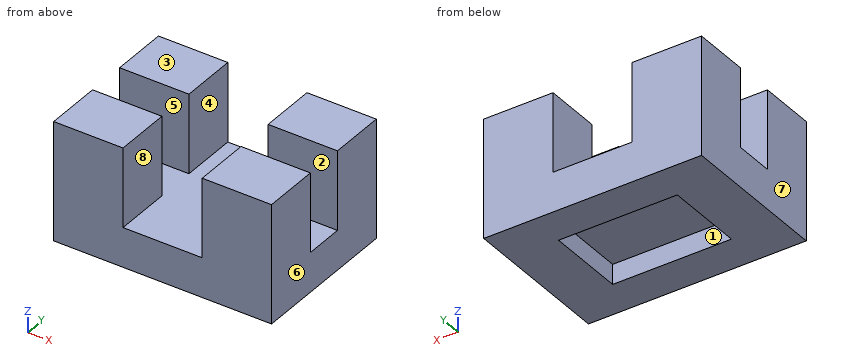
```python
from build123d import *

# Parameters (mm, degrees)
F0_W     = 17.4752
F0_H     = 12.2936
F1_DEPTH = 9.525
F2_W     = 6.35
F2_H     = 12.2936
F3_DEPTH = 6.35
F4_W     = 17.4752
F4_H     = 3.175
F5_DEPTH = 6.35
F6_W     = 9.525
F6_H     = 6.35
F7_DEPTH = 1.6002


with BuildPart() as f1:
    # F0 (on Top) → F1 (new body)
    with BuildSketch(Plane.XY):
        Rectangle(F0_W, F0_H)
    extrude(amount=F1_DEPTH)

    # F2 (on face) → F3 (cut)
    with BuildSketch(Plane.XY.offset(9.525)):
        Rectangle(F2_W, F2_H)
    extrude(amount=-F3_DEPTH, mode=Mode.SUBTRACT)

    # F4 (on face) → F5 (cut)
    with BuildSketch(Plane.XY.offset(9.525)):
        Rectangle(F4_W, F4_H)
    extrude(amount=-F5_DEPTH, mode=Mode.SUBTRACT)

    # F6 (on face) → F7 (cut)
    with BuildSketch(Plane(origin=(0, 0, 0), x_dir=(1, 0, 0), z_dir=(0, 0, -1))):
        Rectangle(F6_W, F6_H)
    extrude(amount=-F7_DEPTH, mode=Mode.SUBTRACT)


solid = f1.part
```
Geometry: final body of the model. Coordinates: model frame, mm. Face numbers are marked on the shaded views. A direction names the side the tool comes from. Round coordinates to 2 decimals unless told otherwise and drop trailing zeros. Write each loop counter-clockwise with the first axis right and the second up, starting at its lowest first coordinate (ties: lowest second). Pieces come first, ordered by that corner, then holes.
Item 1: Set-up query: the marked faces 1, 2, 3 and 4. Return all of +Z, -Z, +X, -X, +Y, -Y with unobstructed straight access to the full face (end or side cutting, diameter ignored); none if empty.
Item 2: Section query B-B (y = 4.5). Return loops of the section in (x, z) (3 decimals).
Item 3: Material intervals for L1, parallel to Y at x = 6, z = 7.25; L2, parallel to X at y = 2.75, z = 6.5 (3 decimals); L3, parallel to X at y = 3, z = 1.25, sorted ascending.
Item 4: Pin query (flat end, axial travel): P1, Ø5, axis at x = 3, y = -4, coming from the +Z side (3 decimals); P2, Ø3.5, axis at x = -1, y = -2, coming from the +Z side (3 decimals); P3, Ø2, axis at x = -0.5, z = 5, coming from the +Y side (1 decimal); P4, Ø1.9, axis at x = 0, y = 0.5, coming from the -Z side. Return the tip coordinate at first contact, or that it passes through.
Item 5: Mould query, pull axis X, two halves, no side actions, for the marked faces 5, 6, 7 and 8. Classes: +X half, -X half, draft (parallel to the pull), parting line (faces both ways), or undercut.
Item 6: Section query C-C (x = 4.5). Return loops of the section in (y, z) (1 decimal), plus the area to 3 significant figures.
Item 7: Section query D-D (y = -0.5). Return loops of the section in (x, z) (1 decimal), plus the area to 3 significant figures.
Item 8: Section query A-A (z = 7). Return loops of the section in (x, y) (1 decimal).
Completed:
1. face 1: -Z
1. face 2: +Z, +X, -X
1. face 3: +Z, +X, -X, +Y, -Y
1. face 4: +Z, +Y, -Y
2. outline: (-8.738, 0) - (8.738, 0) - (8.738, 9.525) - (3.175, 9.525) - (3.175, 3.175) - (-3.175, 3.175) - (-3.175, 9.525) - (-8.738, 9.525) - close
3. L1: y = -6.15 to -1.59, 1.59 to 6.15
3. L2: x = -8.738 to -3.175, 3.175 to 8.738
3. L3: x = -8.74 to -4.76, 4.76 to 8.74
4. P1: stops at z = 9.525
4. P2: stops at z = 3.175
4. P3: passes through
4. P4: stops at z = 1.6
5. face 5: draft
5. face 6: +X half
5. face 7: -X half
5. face 8: undercut
6. outline: (-6.1, 0) - (-3.2, 0) - (-3.2, 1.6) - (3.2, 1.6) - (3.2, 0) - (6.1, 0) - (6.1, 9.5) - (1.6, 9.5) - (1.6, 3.2) - (-1.6, 3.2) - (-1.6, 9.5) - (-6.1, 9.5) - close
6. area: 86.8 mm2
7. outline: (-8.7, 0) - (-4.8, 0) - (-4.8, 1.6) - (4.8, 1.6) - (4.8, 0) - (8.7, 0) - (8.7, 3.2) - (-8.7, 3.2) - close
7. area: 40.2 mm2
8. outline: (-8.7, -6.1) - (-3.2, -6.1) - (-3.2, -1.6) - (-8.7, -1.6) - close; (-8.7, 1.6) - (-3.2, 1.6) - (-3.2, 6.1) - (-8.7, 6.1) - close; (3.2, -6.1) - (8.7, -6.1) - (8.7, -1.6) - (3.2, -1.6) - close; (3.2, 1.6) - (8.7, 1.6) - (8.7, 6.1) - (3.2, 6.1) - close
